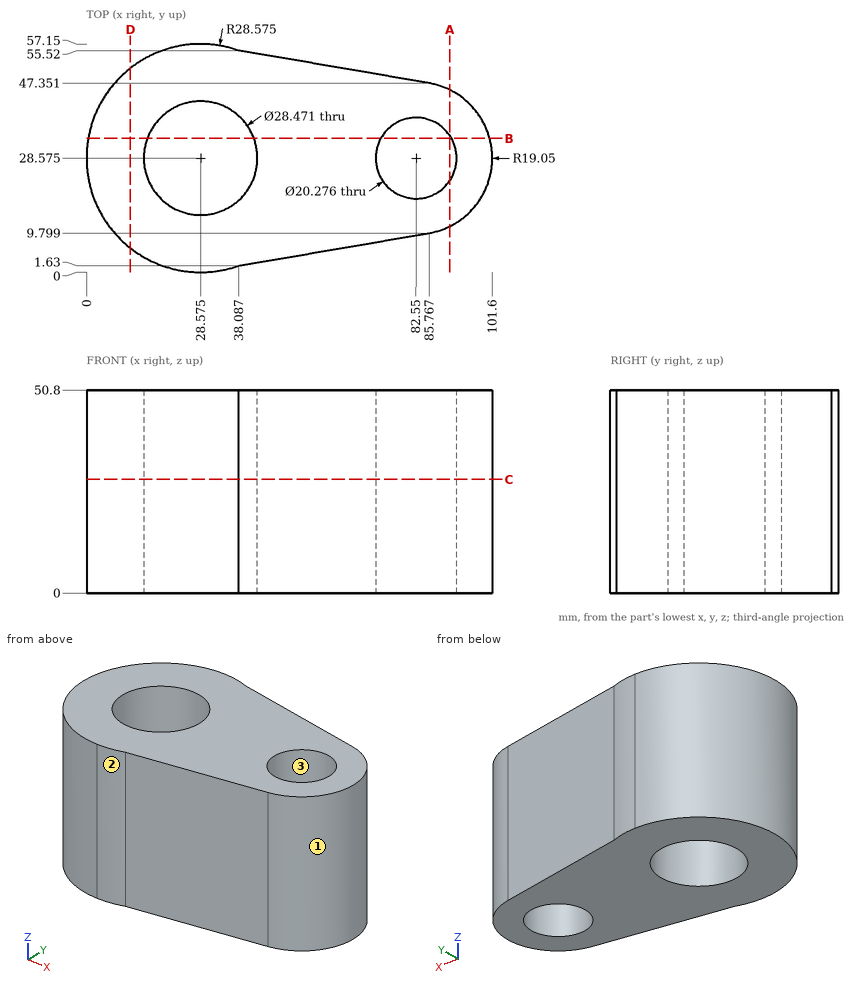
Job drawing, mm, ordinate dimensions from the low corner. One solid piece. Give positions to 0.01 mm unless a question says otherwise; leave off trailing zeros. Loops run counter-clockwise (first coordinate to the right, second up) from the corner with the lowest first, then second, coordinate; pieces in that order, holes last. Notation, with made-up numbers: M 4,-21 L 40,-21 A19 cw 40,-15 Z; hole C -16.5,27.5 d11. An arc over 180 degrees is marked long. Return JSON: item names as keys, results as strings.
1) Saw through at A-A, the plane x = 91. List the corners of the cut face in (y, z).
Calculated:
{"outline": "M 11.5,0 L 22.97,0 L 22.97,50.8 L 11.5,50.8 Z; M 34.18,0 L 45.65,0 L 45.65,50.8 L 34.18,50.8 Z"}
2) Drill centre lines: line 1 (X direction, y = 28.5, z = 34.5); line 2 (Y direction, x = 82.55, z = 19.5); line 3 (Y direction, x = 49.5, z = 17) (1 decimal). Where is each one in solid material? Low to high.
Calculated:
{"line 1": "x = 0 to 14.34, 42.81 to 72.41, 92.69 to 101.6", "line 2": "y = 9.25 to 18.44, 38.71 to 47.9", "line 3": "y = 3.6 to 53.6"}
3) Saw through at D-D, the plane x = 11. List the corners of the cut face in (y, z), then the cut area to 3 significant figures.
Calculated:
{"outline": "M 6.04,0 L 51.11,0 L 51.11,50.8 L 6.04,50.8 Z", "area": "2,290 mm2"}
4) Flat gauge pins, fed straight in: pin 1 Ø6 at (y, z) = (47, 16) entering from +X; pin 2 Ø12 at (x, z) = (39, 22) entering from -Y (1 decimal); pin 3 Ø3 at (x, z) = (77, 28) entering from +Y. Where does each tip first touch, or does it go through?
Calculated:
{"pin 1": "stops at x = 93.73", "pin 2": "stops at y = 0.3", "pin 3": "stops at y = 49.11"}
5) Saw through at C-C, the plane z = 28.5. Count the separate pieces of the cut face and the enclosed holes in it, then the cut area to 3 significant figures.
Calculated:
{"separate pieces": "1", "enclosed holes": "2", "area": "3,480 mm2"}
6) Pull direction Y, two halves, no side cores. Call the marked faces 1, 2 and 3: released by +Y, released by -Y, zero draft, split by the parting line, or undercut.
Calculated:
{"face 1": "split by the parting line", "face 2": "released by -Y", "face 3": "undercut"}
7) Saw through at B-B, the plane y = 33.5. List the corners of the cut face in (x, z).
Calculated:
{"outline": "M 0.43,0 L 15.22,0 L 15.22,50.8 L 0.43,50.8 Z; M 41.93,0 L 73.69,0 L 73.69,50.8 L 41.93,50.8 Z; M 91.41,0 L 100.95,0 L 100.95,50.8 L 91.41,50.8 Z"}
